from build123d import *

# Parameters (mm, degrees)
SKETCH1_W           = 92
SKETCH1_H           = 60
SKETCH1_R           = 3.15
SKETCH1_W_2         = 71
SKETCH1_H_2         = 24
BOSS_EXTRUDE1_DEPTH = 3


with BuildPart() as part:
    # Sketch1 → Boss-Extrude1 (new body)
    with BuildSketch(Plane(origin=(0, 0, 0), x_dir=(1, 0, 0), z_dir=(0, 1, 0))):
        Rectangle(SKETCH1_W, SKETCH1_H)
        with Locations(Location((-26.7, -17.491017964, 0), (0, 0, 270))):
            Circle(SKETCH1_R, mode=Mode.SUBTRACT)
        with Locations(Location((-8.28, -17.491017964, 0), (0, 0, 270))):
            Circle(SKETCH1_R, mode=Mode.SUBTRACT)
        with Locations(Location((10.14, -17.491017964, 0), (0, 0, 270))):
            Circle(SKETCH1_R, mode=Mode.SUBTRACT)
        with Locations(Location((28.56, -17.491017964, 0), (0, 0, 270))):
            Circle(SKETCH1_R, mode=Mode.SUBTRACT)
        with Locations((0, 4.87)):
            Rectangle(SKETCH1_W_2, SKETCH1_H_2, mode=Mode.SUBTRACT)
    extrude(amount=BOSS_EXTRUDE1_DEPTH)


solid = part.part
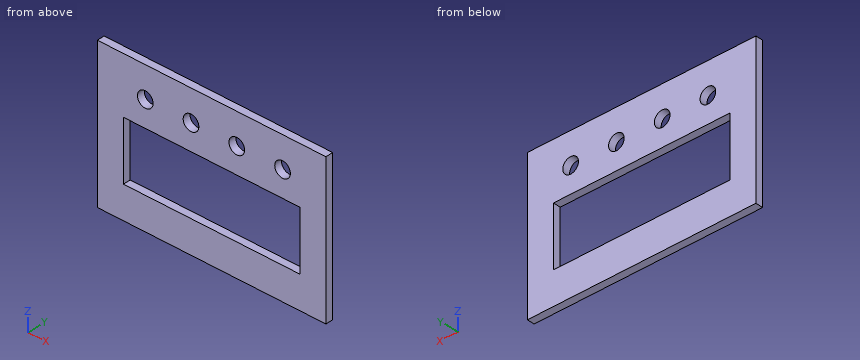
Geometry check sheet. Reference: the model listing, model coordinates, mm. Round coordinates to 2 decimals unless told otherwise and drop trailing zeros. Loops run counter-clockwise (first coordinate to the right, second up) from the corner with the lowest first, then second, coordinate; pieces in that order, holes last.
Item 1: Cross-section at B-B on y = 1.45. Record the boundary of the cut face in (x, z), then the cut area to 3 significant figures.
Item 2: Thickness scan on line 1 (Z direction, x = 18.5, y = 0.4); line 2 (X direction, y = 2, z = -14.5); line 3 (Z direction, x = 8, y = 0.2). Record the ranges inside material, lowest first.
Item 3: Cross-section at A-A on x = 16.5. Record the boundary of the cut face in (y, z).
Answer sheet:
1. outline: (-46, -30) - (46, -30) - (46, 30) - (-46, 30) - close; hole (-35.5, -16.87) - (35.5, -16.87) - (35.5, 7.13) - (-35.5, 7.13) - close; hole circle Ø6.3 at (-26.7, 17.49); hole circle Ø6.3 at (-8.28, 17.49); hole circle Ø6.3 at (10.14, 17.49); hole circle Ø6.3 at (28.56, 17.49)
1. area: 3,690 mm2
2. line 1: z = -30 to -16.87, 7.13 to 30
2. line 2: x = -46 to -35.5, 35.5 to 46
2. line 3: z = -30 to -16.87, 7.13 to 15.18, 19.8 to 30
3. outline: (0, -30) - (3, -30) - (3, -16.87) - (0, -16.87) - close; (0, 7.13) - (3, 7.13) - (3, 30) - (0, 30) - close
